```python
from build123d import *

# Parameters (mm, degrees)
BOSS_EXTRUDE1_DEPTH = 3


with BuildPart() as part:
    # Sketch3 → Boss-Extrude1 (new body)
    with BuildSketch(Plane(origin=(0, 0, 0), x_dir=(1, 0, 0), z_dir=(0, 1, 0))):
        with BuildLine():
            Line((-36.319194267, -89.236860887), (144.478790315, -23.431776084))
            ThreePointArc((144.478790315, -23.431776084), (165.000000077, -19.813332936), (185.52120983, -23.431776136))
            Line((185.52120983, -23.431776136), (366.319192052, -89.236860081))
            ThreePointArc((366.319192052, -89.236860081), (416.877444894, -67.142834059), (397.269838057, -15.569346002))
            Line((397.269838057, -15.569346002), (344.206351456, 9.829836443))
            ThreePointArc((344.206351456, 9.829836443), (333.847680817, 19.053826006), (330, 32.379717841))
            Line((330, 32.379717841), (330, 330))
            Line((330, 330), (0, 330))
            Line((0, 330), (0, 32.379717841))
            ThreePointArc((0, 32.379717841), (-3.847681031, 19.053825667), (-14.206352179, 9.829836096))
            Line((-14.206352179, 9.829836096), (-67.269835876, -15.569344958))
            ThreePointArc((-67.269835876, -15.569344958), (-86.877445819, -67.142831858), (-36.319194267, -89.236860887))
        make_face()
    extrude(amount=BOSS_EXTRUDE1_DEPTH)


solid = part.part
```
Verification items for the finished model (mm, model axes). Coordinates: 2 decimals unless noted, no trailing zeros. Order: outer loops, then holes, each group sorted by start corner. A loop starts at its lowest first (then second) coordinate and runs counter-clockwise, first axis right, second up. Notation, with made-up numbers: (-31, -35) - (3, -35) arc R10 ccw to (3, -18) - close; hole circle Ø8 at (-30.5, 10.25). An arc over 180 degrees is marked (long way). Return JSON: item names as keys, results as strings.
(1) Section check B-B, the plane y = 0.75. Record the cut outline in (x, z).
Filled sheet:
{"outline": "(-67.27, 15.57) - (-14.21, -9.83) arc R25 cw to (0, -32.38) - (0, -330) - (330, -330) - (330, -32.38) arc R25 cw to (344.21, -9.83) - (397.27, 15.57) arc R40 ccw to (366.32, 89.24) - (185.52, 23.43) arc R60 cw to (144.48, 23.43) - (-36.32, 89.24) arc R40 ccw to start"}
(2) Thickness scan on line 1 along X through (y, z) = (2.45, -218); line 2 along Z through (x, y) = (217.5, 1.7); line 3 along Z through (x, y) = (209, 0.6). Record the ranges inside material, lowest first.
Filled sheet:
{"line 1": "x = 0 to 330", "line 2": "z = -330 to 35.07", "line 3": "z = -330 to 31.98"}
(3) Go/stop test with flat-tipped pins: pin 1 (1 mm diameter, centred on y = 2, z = -45.5, fed in from -X); pin 2 (1.5 mm diameter, centred on y = 0.5, z = -141.5, fed in from +X); pin 3 (1 mm diameter, centred on x = -3, y = 1, fed in from -Z). Record where each tip stops, or that it passes through.
Filled sheet:
{"pin 1": "stops at x = 0", "pin 2": "stops at x = 330", "pin 3": "stops at z = -21.48"}
(4) Mould release check, pull along X, two halves, no side actions. Record for faces 1 (the flat face through (275, 1, 56)), 2 (the flat face through (161, 3, -122)), 3 (the flat face through (-40.367, 1.479, 2.692)), 4 (the flat face through (52.8, 1.5, 56.8)): pulls with the +X half, pulls with the -X half, needs draft (parallel to the pull), parting line crosses it, or undercut.
Filled sheet:
{"face 1": "undercut", "face 2": "needs draft", "face 3": "pulls with the -X half", "face 4": "undercut"}
(5) Section check A-A, the plane z = 40. Record the cut outline in (x, y).
Filled sheet:
{"outline": "(-88.27, 0) - (98.96, 0) - (98.96, 3) - (-88.27, 3) - close; (231.04, 0) - (418.27, 0) - (418.27, 3) - (231.04, 3) - close"}
(6) Section check D-D, the plane x = 101. Record the cut outline in (y, z), and give its area (3 significant figures).
Filled sheet:
{"outline": "(0, -330) - (3, -330) - (3, 39.26) - (0, 39.26) - close", "area": "1,110 mm^2"}
(7) Section check C-C, the plane z = -176. Record the cut outline in (x, y), and give its area (3 significant figures).
Filled sheet:
{"outline": "(0, 0) - (330, 0) - (330, 3) - (0, 3) - close", "area": "990 mm^2"}
